from build123d import *

# Parameters (mm, degrees)
F0_W     = 14
F0_H     = 3
F0_W_2   = 3
F1_DEPTH = 20
F2_DEPTH = 3
F3_W     = 3
F3_H     = 3
F4_DEPTH = 100
F5_W     = 3
F5_H     = 3.5
F6_DEPTH = 100
F7_R     = 1.5


with BuildPart() as f1:
    # F0 (on Front) → F1 (new body)
    with BuildSketch(Plane.XZ):
        Polygon((10, 1.5), (10, 4.5), (-10, 4.5), (-10, 1.5), (-7, 1.5), (7, 1.5), align=None)
        Rectangle(F0_W, F0_H)
        with Locations((11.5, 0)):
            Rectangle(F0_W_2, F0_H)
        with Locations((8.5, 0)):
            Rectangle(F0_W_2, F0_H)
        with Locations((-8.5, 0)):
            Rectangle(F0_W_2, F0_H)
        Polygon((10, -4.5), (10, -1.5), (7, -1.5), (-7, -1.5), (-10, -1.5), (-10, -4.5), align=None)
    extrude(amount=-F1_DEPTH)

    # F0 (on Front) → F2 (join)
    with BuildSketch(Plane.XZ):
        with Locations((-8.5, 0)):
            Rectangle(F0_W_2, F0_H)
        Rectangle(F0_W, F0_H)
        with Locations((8.5, 0)):
            Rectangle(F0_W_2, F0_H)
        with Locations((11.5, 0)):
            Rectangle(F0_W_2, F0_H)
    extrude(amount=F2_DEPTH)

    # F3 (on face) → F4 (cut)
    with BuildSketch(Plane.YZ.offset(13)):
        Polygon((23, -1.75), (23, 1.75), (17, 1.75), (17, 1.5), (20, 1.5), (20, -1.5), (17, -1.5), (17, -1.75), align=None)
        with Locations((18.5, 0)):
            Rectangle(F3_W, F3_H)
    extrude(amount=-F4_DEPTH, mode=Mode.SUBTRACT)

    # F5 (on face) → F6 (cut)
    with BuildSketch(Plane(origin=(0, 17, 0), x_dir=(-1, 0, 0), z_dir=(0, 1, 0))):
        with Locations((11.5, 0)):
            Rectangle(F5_W, F5_H)
        with Locations((8.5, 0)):
            Rectangle(F5_W, F5_H)
    extrude(amount=-F6_DEPTH, mode=Mode.SUBTRACT)

    # F7
    f7_edges = [f1.edges().sort_by_distance(p)[0] for p in [
        (-7, -3, 0),
        (13, -3, 0),
        (10, 0, 3),
        (10, 0, -3),
        (-10, 0, -3.125),
        (-10, 0, 3.125),
        (-7, 17, 0),
        (-10, 20, 3.125),
        (-10, 20, -3.125),
        (13, 17, 0),
        (10, 20, 3.125),
        (10, 20, -3.125),
    ]]
    fillet(f7_edges, radius=F7_R)


solid = f1.part
Check sheet for the modelled part. Datum: model origin and axes. Units: mm. A direction names the side the tool comes from. Round coordinates to 2 decimals unless told otherwise and drop trailing zeros. Loops run counter-clockwise (first coordinate to the right, second up) from the corner with the lowest first, then second, coordinate; pieces in that order, holes last. Notation, with made-up numbers: (-30.75, 31.25) -> (18.25, 31.25) arc R28 cw to (18.25, 56.25) -> close; hole circle Ø4 at (36.5, 1.25). An arc over 180 degrees is marked (long way). Put each result on its own line as item: value. Start each with the question number.
1. Section check B-B (x = -0.75). Enter the section's corners in (y, z), plus the area to 4 significant figures.
2. Section check A-A (y = 18). Enter the section's corners in (x, z), plus the area to 3 significant figures.
3. Scan lines: probe 1 along X at (y, z) = (11, -0.5); probe 2 along Y at (x, z) = (-4.5, -2); probe 3 along X at (y, z) = (14.5, 2.75). Record each from-to range of solid material in increasing order.
4. Access from +Z, -Z, +X, -X, +Y, -Y to the whole of each face (thin tool, end or side, straight path). Record for faces 1 (the face through (10, 10, -3)), 2 (the face through (0, 0, -3)), 3 (the face through (3, 17, 0)).
5. Gauge pin test, flat ends, axial feed: pin 1 (2.5 mm diameter, centred on y = 6, z = 3, fed in from +X); pin 2 (1.8 mm diameter, centred on x = 1.5, z = -0.5, fed in from +Y); pin 3 (2.5 mm diameter, centred on x = 2, z = -3.5, fed in from -Y). Record the tip position at first contact, or that the pin passes through.
6. Section check C-C (z = 2.25). Enter the section's corners in (x, y).
7. Draft check along Z on faces 4 (the face through (0, 20, -3)), 5 (the face through (-7, 7, 0)), 6 (the face through (6.8, -0.4, 1.5)). Enter one of: +Z half, -Z half, draft (parallel to the pull), parting line (faces both ways), or undercut.
8. Section check D-D (y = 9.75). Enter the section's corners in (x, z).
Findings:
1. outline: (-3, -1.5) -> (0, -1.5) -> (0, -4.5) -> (20, -4.5) -> (20, -1.75) -> (17, -1.75) -> (17, 1.75) -> (20, 1.75) -> (20, 4.5) -> (0, 4.5) -> (0, 1.5) -> (-3, 1.5) -> close
1. area: 178.5 mm^2
2. outline: (-10, -4.5) -> (10, -4.5) -> (10, -1.75) -> (-10, -1.75) -> close; (-10, 1.75) -> (10, 1.75) -> (10, 4.5) -> (-10, 4.5) -> close
2. area: 110 mm^2
3. probe 1: x = -7 to 13
3. probe 2: y = 0 to 20
3. probe 3: x = -10 to 10
4. face 1: -Z, +X, +Y, -Y
4. face 2: -Z, +X, -X, -Y
4. face 3: +X, -X, +Y
5. pin 1: stops at x = 10
5. pin 2: stops at y = 17
5. pin 3: stops at y = 0
6. outline: (-10, 1.5) arc R1.5 ccw to (-8.5, 0) -> (8.5, 0) arc R1.5 ccw to (10, 1.5) -> (10, 18.5) arc R1.5 ccw to (8.5, 20) -> (-8.5, 20) arc R1.5 ccw to (-10, 18.5) -> close
7. face 4: draft
7. face 5: undercut
7. face 6: +Z half
8. outline: (-10, -4.5) -> (10, -4.5) -> (10, -1.5) -> (13, -1.5) -> (13, 1.5) -> (10, 1.5) -> (10, 4.5) -> (-10, 4.5) -> (-10, 1.75) -> (-7, 1.75) -> (-7, -1.75) -> (-10, -1.75) -> close
